The model under review builds one solid part; all positions refer to its coordinate system, in mm. A direction names the side the tool comes from. Round coordinates to 2 decimals unless told otherwise and drop trailing zeros. Loops run counter-clockwise (first coordinate to the right, second up) from the corner with the lowest first, then second, coordinate; pieces in that order, holes last. Notation, with made-up numbers: (30, 77.25) -> (41, 77.25) arc R18 cw to (41, 86.25) -> close; hole circle Ø5 at (-22, 20). An arc over 180 degrees is marked (long way). Return JSON: item names as keys, results as strings. Group by question number.
```python
from build123d import *

# Parameters (mm, degrees)
F1_DEPTH = 109.474
F2_W     = 37.3121537268
F2_H     = 12.854102999
F2_R     = 7.6049065211
F3_DEPTH = 155.1973314414
F4_W     = 59.8052963614
F4_H     = 28.047692441
F5_DEPTH = 66.7983458767
F6_W     = 56.3981542364
F6_H     = 109.474
F7_DEPTH = 7.112


with BuildPart() as f1:
    # F0 (on Front) → F1 (new body)
    with BuildSketch(Plane.XZ):
        Polygon((-48.026971519, 66.7973458767), (-48.026971519, 0), (107.1693599224, 0), (39.2185337842, 66.7973458767), align=None)
    extrude(amount=F1_DEPTH)

    # F2 (on face) → F3 (cut, through all)
    with BuildSketch(Plane(origin=(-48.026971519, 0, 0), x_dir=(0, -1, 0), z_dir=(-1, 0, 0))):
        with Locations((53.3815380186, 60.3702943772)):
            Rectangle(F2_W, F2_H)
        with Locations((30.8165661991, 42.21656546)):
            Circle(F2_R)
        with Locations((31.5272733569, 20.5399803817)):
            Circle(F2_R)
        with Locations((64.8002144327, 20.1804041862)):
            Circle(F2_R)
        with Locations((65.5109215906, 41.8569892645)):
            Circle(F2_R)
    extrude(amount=-F3_DEPTH, mode=Mode.SUBTRACT)

    # F4 (on face) → F5 (cut, through all)
    with BuildSketch(Plane(origin=(0, 0, 0), x_dir=(1, 0, 0), z_dir=(0, 0, -1))):
        with Locations((77.2667117417, 95.4501537795)):
            Rectangle(F4_W, F4_H)
    extrude(amount=-F5_DEPTH, mode=Mode.SUBTRACT)

    # F6 (on face) → F7 (cut)
    with BuildSketch(Plane(origin=(0, 0, 0), x_dir=(1, 0, 0), z_dir=(0, 0, -1))):
        with Locations((-19.8278944008, 54.737)):
            Rectangle(F6_W, F6_H)
    extrude(amount=-F7_DEPTH, mode=Mode.SUBTRACT)


solid = f1.part
```
1. We need section D-D, the plane x = 1. Write out the cut boundary in (y, z).
2. We need section C-C, the plane z = 46. Write out the cut boundary in (x, y), then the cut area to 3 significant figures.
3. Wall thickness on line 1 (Y direction, x = -33, z = 20.5); line 2 (Z direction, x = -26, y = -25.5); line 3 (Z direction, x = -40.5, y = -66.5): over which ranges is each line inside the solid? List them lowest first.
4. We need section A-A, the plane y = -61.5. Write out the cut boundary in (x, z).
5. We need section B-B, the plane z = 63. Write out the cut boundary in (x, y).
6. For P1, Ø4, axis at x = -12, y = -65.5, coming from the -Z side; P2, Ø11, axis at x = -22.5, y = -53, coming from the +Z side; P3, Ø1.5, axis at y = -23.5, z = 18.5, coming from the +X side; P4, Ø17.5, axis at y = -64.8, z = 20.18, coming from the -X side, all flat-tipped, find the tip position at first contact; note any pin that passes through.
7. Tool access review of faces 4 (the face through (22.269, -63.152, 12.756)), 5 (the face through (-48.027, -54, 37)), 6 (the face through (47.364, -95, 29)), 7 (the face through (1, -53, 53.943)), 8 (the face through (-20, -56, 7.112)): name each direction out of +Z, -Z, +X, -X, +Y, -Y from which nothing blocks a thin tool from reaching the whole face with its end or side.
8. Draft analysis for pull direction Y (two halves, no side actions). For faces 1 (the face through (73.7, -41.8, 32.9)), 2 (the face through (11, 0, 34)), 3 (the face through (22.089, -29.879, 13.116)), state which applies: pulls with the +Y half, pulls with the -Y half, needs draft (parallel to the pull), parting line crosses it, or undercut.
Check sheet entries:
{
 "1": {"outline": "(-109.47, 7.11) -> (0, 7.11) -> (0, 66.8) -> (-34.73, 66.8) -> (-34.73, 53.94) -> (-72.04, 53.94) -> (-72.04, 66.8) -> (-109.47, 66.8) -> close; hole circle Ø15.21 at (-65.51, 41.86); hole circle Ø15.21 at (-64.8, 20.18); hole circle Ø15.21 at (-31.53, 20.54); hole circle Ø15.21 at (-30.82, 42.22)"},
 "2": {"outline": "(-48.03, -109.47) -> (47.36, -109.47) -> (47.36, -81.43) -> (60.38, -81.43) -> (60.38, -71.89) -> (-48.03, -71.89) -> close; (-48.03, -59.13) -> (60.38, -59.13) -> (60.38, -37.41) -> (-48.03, -37.41) -> close; (-48.03, -24.22) -> (60.38, -24.22) -> (60.38, 0) -> (-48.03, 0) -> close", "area": "8,690 mm²"},
 "3": {"line 1": "y = -109.47 to -72.4, -57.2 to -39.13, -23.92 to 0", "line 2": "z = 7.11 to 15.9, 25.18 to 36.78, 47.65 to 66.8", "line 3": "z = 7.11 to 12.77, 27.59 to 34.32, 49.4 to 53.94"},
 "4": {"outline": "(-48.03, 7.11) -> (8.37, 7.11) -> (8.37, 0) -> (107.17, 0) -> (93.61, 13.33) -> (-48.03, 13.33) -> close; (-48.03, 27.03) -> (79.67, 27.03) -> (71.16, 35.4) -> (-48.03, 35.4) -> close; (-48.03, 48.32) -> (58.02, 48.32) -> (52.29, 53.94) -> (-48.03, 53.94) -> close"},
 "5": {"outline": "(-48.03, -109.47) -> (43.08, -109.47) -> (43.08, -72.04) -> (-48.03, -72.04) -> close; (-48.03, -34.73) -> (43.08, -34.73) -> (43.08, 0) -> (-48.03, 0) -> close"},
 "6": {"P1": "stops at z = 7.11", "P2": "stops at z = 53.94", "P3": "stops at x = 89.11", "P4": "stops at x = -48.03"},
 "7": {"face 4": "+X, -X", "face 5": "+Z, -Z, -X, +Y, -Y", "face 6": "+Z, -Z, +X, -Y", "face 7": "+Z, +X, -X", "face 8": "-Z, -X, +Y, -Y"},
 "8": {"face 1": "needs draft", "face 2": "pulls with the +Y half", "face 3": "undercut"}
}
